```python
from build123d import *
from build123d.topology import SkipClean

# Parameters (mm, degrees)
ESBO_O1_R                            = 20
RESSALTO_EXTRUS_O2_DEPTH             = 20
RESSALTO_EXTRUS_O3_DEPTH             = 10
RESSALTO_EXTRUS_O3_DIRECTION_2_REACH = 42.62
CORTE_EXTRUS_O2_START                = -12.5
CORTE_EXTRUS_O2_DEPTH                = 12.5


with BuildPart() as part:
    # Esboço1 → Ressalto-extrusão2 (new body)
    with BuildSketch(Plane(origin=(0, 0, 0), x_dir=(1, 0, 0), z_dir=(0, 1, 0))):
        with BuildLine():
            ThreePointArc((-12.5, -21.650635095), (0, -25), (12.5, -21.650635095))
            ThreePointArc((12.5, -21.650635095), (21.650635095, -12.5), (25, 0))
            ThreePointArc((25, 0), (-12.5, 21.650635095), (-12.5, -21.650635095))
        make_face()
        with Locations(Location((0, 0, 0), (0, 0, 270))):
            Circle(ESBO_O1_R, mode=Mode.SUBTRACT)
    extrude(amount=RESSALTO_EXTRUS_O2_DEPTH)

    # Esboço2 → Ressalto-extrusão3 (add)
    with BuildSketch(Plane(origin=(0, 20, 0), x_dir=(1, 0, 0), z_dir=(0, 1, 0))):
        with BuildLine():
            Line((-12.5, -15.612494996), (-12.5, -12.951833847))
            ThreePointArc((-12.5, -12.951833847), (0, 18), (12.5, -12.951833847))
            Line((12.5, -12.951833847), (12.5, -15.612494996))
            ThreePointArc((12.5, -15.612494996), (0, 20), (-12.5, -15.612494996))
        make_face()
    extrude(amount=RESSALTO_EXTRUS_O3_DEPTH)

    # Ressalto-extrusão3 direction 2: up to this face of the body (flat: up to its plane)
    ressalto_extrus_o3_direction_2_end = Plane(part.part.faces().sort_by_distance((12.146446609, 0, -21.038262659))[0])
    # Esboço2 → Ressalto-extrusão3 direction 2 (add, up to the picked face)
    with BuildSketch(Plane(origin=(0, 20, 0), x_dir=(1, 0, 0), z_dir=(0, 1, 0)), mode=Mode.PRIVATE) as ressalto_extrus_o3_direction_2_sk1:
        with BuildLine():
            Line((-12.5, -15.612494996), (-12.5, -12.951833847))
            ThreePointArc((-12.5, -12.951833847), (0, 18), (12.5, -12.951833847))
            Line((12.5, -12.951833847), (12.5, -15.612494996))
            ThreePointArc((12.5, -15.612494996), (0, 20), (-12.5, -15.612494996))
        make_face()
    ressalto_extrus_o3_direction_2_tool1 = split(extrude(ressalto_extrus_o3_direction_2_sk1.sketch, amount=-RESSALTO_EXTRUS_O3_DIRECTION_2_REACH, mode=Mode.PRIVATE), bisect_by=ressalto_extrus_o3_direction_2_end, keep=Keep.BOTH, mode=Mode.PRIVATE)
    add(ressalto_extrus_o3_direction_2_tool1.solids().sort_by(Axis((13.03556, 20, 14.282164), (0, -1, 0)))[0])

    # Esboço3 → Corte-extrusão2 (cut)
    with SkipClean():  # the faces are left unmerged after this step: merging them gives an invalid solid
        with BuildSketch(Plane(origin=(0, 20, 0), x_dir=(1, 0, 0), z_dir=(0, 1, 0)).offset(CORTE_EXTRUS_O2_START)):
            with BuildLine():
                Line((-18.33030278, 17), (-14.664242224, 13.6))
                ThreePointArc((-14.664242224, 13.6), (19.945337297, 1.477673891), (-12.5, -15.612494996))
                Line((-12.5, -15.612494996), (-12.5, -21.650635095))
                ThreePointArc((-12.5, -21.650635095), (10, -22.912878475), (24.374507866, -5.557280474))
                Line((24.374507866, -5.557280474), (21.773974537, -3.145478163))
                ThreePointArc((21.773974537, -3.145478163), (17.493290141, 13.341094409), (2.726342097, 21.830415909))
                Line((2.726342097, 21.830415909), (3.098116019, 24.807290806))
                ThreePointArc((3.098116019, 24.807290806), (-8.558231465, 23.489501361), (-18.33030278, 17))
            make_face()
        extrude(amount=CORTE_EXTRUS_O2_DEPTH, mode=Mode.SUBTRACT)


solid = part.part
```
Verification items for the finished model (mm, model axes). A direction names the side the tool comes from. Coordinates: 2 decimals unless noted, no trailing zeros. Write each loop counter-clockwise with the first axis right and the second up, starting at its lowest first coordinate (ties: lowest second). Pieces come first, ordered by that corner, then holes. Notation, with made-up numbers: (66, -26.75) - (107, -26.75) arc R18 cw to (107, -13.75) - close; hole circle Ø2 at (35, 7). An arc over 180 degrees is marked (long way). One line per question, with ' | ' between items. Start each with the question number.
1. Section check C-C (z = 16.5). Enter the section's corners in (x, y), plus the area to 3 significant figures.
2. Draft check along X on faces 1 (the flat face through (-0.1, 0, -18.4)), 2 (the flat face through (-12.5, 15, 16)), 3 (the flat face through (23.092, 13.662, 4.368)), 4 (the flat face through (2.91, 13.66, -23.3)). Enter one of: released by +X, released by -X, zero draft, split by the parting line, or undercut.
3. Material ranges on line 1 along Z through (x, y) = (0, 7); line 2 along X through (y, z) = (2.75, 11.5); line 3 along Z through (x, y) = (0, 8.5), recorded low to high.
4. Section check B-B (y = 12.25). Enter the section's corners in (x, z), plus the area to 3 significant figures.
5. Section check D-D (x = 13.5). Enter the section's corners in (y, z), plus the area to 3 significant figures.
6. Section check A-A (x = 0). Enter the section's corners in (y, z).
7. Gauge pin test, flat ends, axial feed: P1, Ø1, axis at x = 18, y = 8.5, coming from the -Z side; P2, Ø9.5, axis at y = 20.5, z = 16.5, coming from the +X side; P3, Ø3, axis at y = 18, z = 14, coming from the -X side; P4, Ø21.5, axis at x = 5, z = -4.5, coming from the +Y side. Record the tip position at first contact, or that the pin passes through.
8. Access from +Z, -Z, +X, -X, +Y, -Y to the whole of each face (thin tool, end or side, straight path). Record for faces 5 (the cylindrical face through (17.641, 13.662, -13.146)), 6 (the flat face through (-16.5, 13.7, -15.3)), 7 (the flat face through (18, 20, -13)), 8 (the cylindrical face through (0, 4, 20)), 9 (the flat face through (-20.2, 20, 2.1)).
Computed values:
1) outline: (-18.78, 0) - (-11.3, 0) - (-11.3, 7.5) - (-12.5, 7.5) - (-12.5, 20) - (-18.78, 20) - close; (11.3, 0) - (18.78, 0) - (18.78, 7.5) - (11.3, 7.5) - close | area: 191 mm²
2) face 1: zero draft | face 2: undercut | face 3: undercut | face 4: released by -X
3) line 1: -25 to -18, 20 to 25 | line 2: -22.2 to -13.85, 13.85 to 22.2 | line 3: -20 to -18
4) outline: (-18.33, -17) - (-14.66, -13.6) arc R20 ccw (long way) to (12.5, 15.61) - (12.5, 12.95) arc R18 cw (long way) to (-12.5, 12.95) - (-12.5, 21.65) arc R25 ccw to start; (2.73, -21.83) - (3.1, -24.81) arc R25 ccw to (24.37, 5.56) - (21.77, 3.15) arc R22 cw to start | area: 494 mm²
5) outline: (0, -21.04) - (20, -21.04) - (20, -17.37) - (7.5, -17.37) - (7.5, -14.76) - (30, -14.76) - (30, -11.91) - (0, -11.91) - close; (0, 11.91) - (30, 11.91) - (30, 14.76) - (7.5, 14.76) - (7.5, 21.04) - (0, 21.04) - close | area: 311 mm²
6) outline: (0, -25) - (7.5, -25) - (7.5, -20) - (30, -20) - (30, -18) - (0, -18) - close; (0, 20) - (7.5, 20) - (7.5, 25) - (0, 25) - close
7) P1: z = -17.85 | P2: x = 16.18 | P3: x = -21.65 | P4: through
8) face 5: +Y | face 6: -Z, +Y | face 7: -Z, +X, +Y | face 8: +Y, -Y | face 9: -X, +Y
